Can you work these out from the model? Positions are in its coordinate system, mm. A direction names the side the tool comes from. Give positions to 0.01 mm unless a question says otherwise; leave off trailing zeros. Write each loop counter-clockwise with the first axis right and the second up, starting at its lowest first coordinate (ties: lowest second). Pieces come first, ordered by that corner, then holes. Notation, with made-up numbers: (21, 35.5) -> (55, 35.5) arc R34 cw to (55, 74.5) -> close; hole circle Ø2 at (57, -14.5). An arc over 180 degrees is marked (long way). Answer as CSV lines item,"result". Start each with the question number.
1. If we section it at B-B on z = -1: Write out the boundary of the cut face in (x, y).
2. If we section it at A-A on x = 2.5: Write out the boundary of the cut face in (y, z).
3. I'm going to push flat-ended pins straight in: P1, Ø5.5, axis at x = -15.88, z = 16.47, coming from the -Y side; P2, Ø4.5, axis at y = -48, z = 5, coming from the +X side. Where does each tip first touch, or does it pass through?
4. On a 3-axis mill with a long thin cutter (end or side, diameter ignored), from which of +Z, -Z, +X, -X, +Y, -Y can I reach the whole of each face in a straight line? I mean faces 4 (the face through (-21, -49, -3.529)), 5 (the face through (-6, 0, 7)), 6 (the face through (-16, -49, 8.971)), 7 (the face through (19, -49, 6.471)). Say none if no direction works.
5. I need wall thicknesses on line 1 (X direction, y = -39.5, z = -5.5); line 2 (Z direction, x = 6.5, y = -31.5); line 3 (Z direction, x = 14.5, y = -10). Which ranges of each line are inside material? Lowest first, please. Write a range as [from, to].
6. If we section it at C-C on x = -17: Write out the boundary of the cut face in (y, z), plus the area to 3 significant figures.
7. If we mould it in two halves opening along Z, with no side actions, what happens to faces 1 (the face through (-6, -100, 7)), 2 (the face through (-18.382, -49, -5)), 3 (the face through (13, -49, -21.029))? For each: pulls with the +Z half, pulls with the -Z half, needs draft (parallel to the pull), parting line crosses it, or undercut.
8. If we section it at D-D on z = 15: Write out the boundary of the cut face in (x, y), plus the area to 3 significant figures.
```python
from build123d import *

# Parameters (mm, degrees)
F0_R     = 4.5
F0_R_2   = 6
F1_DEPTH = 100
F2_R     = 1
F3_R     = 0.5
F4_SIZE  = 0.5


with BuildPart() as f1:
    # F0 (on Front) → F1 (new body)
    with BuildSketch(Plane.XZ):
        Polygon((4.117647, -21.029412), (21.617647, -21.029412), (21.617647, -3.529412), (16.617647, -3.529412), (16.617647, -6.029412), (11.617647, -6.029412), (11.617647, 8.970588), (16.617647, 8.970588), (16.617647, 6.470588), (21.617647, 6.470588), (21.617647, 23.970588), (4.117647, 23.970588), (4.117647, 18.970588), (6.617647, 18.970588), (6.617647, 13.970588), (-8.382353, 13.970588), (-8.382353, 18.970588), (-5.882353, 18.970588), (-5.882353, 23.970588), (-23.382353, 23.970588), (-23.382353, 6.470588), (-18.382353, 6.470588), (-18.382353, 8.970588), (-13.382353, 8.970588), (-13.382353, -6.029412), (-18.382353, -6.029412), (-18.382353, -3.529412), (-23.382353, -3.529412), (-23.382353, -21.029412), (-5.882353, -21.029412), (-5.882353, -16.029412), (-8.382353, -16.029412), (-8.382353, -11.029412), (6.617647, -11.029412), (6.617647, -16.029412), (4.117647, -16.029412), align=None)
        with Locations((-15.882353, -13.529412)):
            Circle(F0_R, mode=Mode.SUBTRACT)
        with Locations((14.117647, -13.529412)):
            Circle(F0_R, mode=Mode.SUBTRACT)
        with Locations((-0.882353, 1.470588)):
            Circle(F0_R_2, mode=Mode.SUBTRACT)
        with Locations((-15.882353, 16.470588)):
            Circle(F0_R, mode=Mode.SUBTRACT)
        with Locations((14.117647, 16.470588)):
            Circle(F0_R, mode=Mode.SUBTRACT)
    extrude(amount=F1_DEPTH)

    # F2
    f2_edges = [f1.edges().sort_by_distance(p)[0] for p in [
        (21.617647, -50, 23.970588),
        (21.617647, -50, -21.029412),
        (-23.382353, -50, -21.029412),
        (-23.382353, -50, 23.970588),
    ]]
    fillet(f2_edges, radius=F2_R)

    # F3
    f3_edges = [f1.edges().sort_by_distance(p)[0] for p in [
        (4.117647, -50, -16.029412),
        (16.617647, -50, 6.470588),
        (16.617647, -50, -3.529412),
        (4.117647, -50, 18.970588),
        (-5.882353, -50, 18.970588),
        (-18.382353, -50, 6.470588),
        (-18.382353, -50, -3.529412),
        (-5.882353, -50, -16.029412),
    ]]
    fillet(f3_edges, radius=F3_R)

    # F4
    f4_edges = [f1.edges().sort_by_distance(p)[0] for p in [
        (-23.382353, -50, -3.529412),
        (-23.382353, -50, 6.470588),
        (-5.882353, -50, 23.970588),
        (4.117647, -50, 23.970588),
        (21.617647, -50, -3.529412),
        (4.117647, -50, -21.029412),
        (21.617647, -50, 6.470588),
        (-5.882353, -50, -21.029412),
    ]]
    chamfer(f4_edges, length=F4_SIZE)


solid = f1.part
```
Computed values:
1,outline,"(-13.38, -100) -> (-6.35, -100) -> (-6.35, 0) -> (-13.38, 0) -> close; (4.59, -100) -> (11.62, -100) -> (11.62, 0) -> (4.59, 0) -> close"
2,outline,"(-100, -11.03) -> (0, -11.03) -> (0, -3.49) -> (-100, -3.49) -> close; (-100, 6.43) -> (0, 6.43) -> (0, 13.97) -> (-100, 13.97) -> close"
3,P1,"passes through"
3,P2,"stops at x = 21.62"
4,face 4,"-X, +Y, -Y"
4,face 5,"+Z, -Z, +X, -X, +Y"
4,face 6,"+Y, -Y"
4,face 7,"+X, +Y, -Y"
5,line 1,"x = [-23.38, -18.38], [-13.38, 11.62], [16.62, 21.62]"
5,line 2,"z = [-21.03, -16.03], [-11.03, 13.97], [18.97, 23.97]"
5,line 3,"z = [-21.03, -18.01], [-9.05, -6.03], [8.97, 11.99], [20.95, 23.97]"
6,outline,"(-100, -21.03) -> (0, -21.03) -> (0, -17.89) -> (-100, -17.89) -> close; (-100, -9.17) -> (0, -9.17) -> (0, -6.03) -> (-100, -6.03) -> close; (-100, 8.97) -> (0, 8.97) -> (0, 12.11) -> (-100, 12.11) -> close; (-100, 20.83) -> (0, 20.83) -> (0, 23.97) -> (-100, 23.97) -> close"
6,area,"1,260 mm2"
7,face 1,"needs draft"
7,face 2,"undercut"
7,face 3,"pulls with the -Z half"
8,outline,"(-23.38, -100) -> (-20.14, -100) -> (-20.14, 0) -> (-23.38, 0) -> close; (-11.63, -100) -> (-8.38, -100) -> (-8.38, 0) -> (-11.63, 0) -> close; (6.62, -100) -> (9.86, -100) -> (9.86, 0) -> (6.62, 0) -> close; (18.37, -100) -> (21.62, -100) -> (21.62, 0) -> (18.37, 0) -> close"
8,area,"1,300 mm2"
